For this review, take the finished solid that the model builds, in its own axes (mm). Face numbers are marked on the shaded views. Give positions to 0.01 mm unless a question says otherwise; leave off trailing zeros. Write each loop counter-clockwise with the first axis right and the second up, starting at its lowest first coordinate (ties: lowest second). Pieces come first, ordered by that corner, then holes. Notation, with made-up numbers: M 23,51 L 38,51 A21 ccw 38,76 Z; hole C 14,58 d3. An arc over 180 degrees is marked long. Write item = value, one per line.
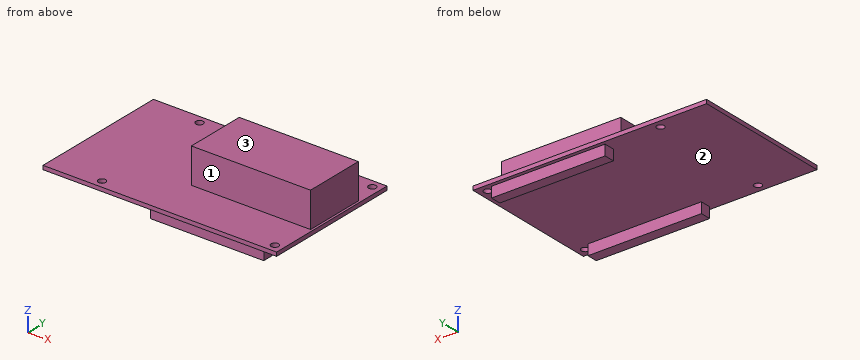
```python
from build123d import *

# Parameters (mm, degrees)
F0_W     = 100
F0_H     = 60
F0_R     = 1.6
F1_DEPTH = 1.65
F2_W     = 48.6
F2_H     = 4.5
F3_DEPTH = 4.5
F4_W     = 51
F4_H     = 26
F5_DEPTH = 15


with BuildPart() as f1:
    # F0 (on Top) → F1 (new body)
    with BuildSketch(Plane.XY):
        Rectangle(F0_W, F0_H)
        with Locations((-27.5, -26.5)):
            Circle(F0_R, mode=Mode.SUBTRACT)
        with Locations((46.5, -26.5)):
            Circle(F0_R, mode=Mode.SUBTRACT)
        with Locations((-27.5, 26.5)):
            Circle(F0_R, mode=Mode.SUBTRACT)
        with Locations((46.5, 26.5)):
            Circle(F0_R, mode=Mode.SUBTRACT)
    extrude(amount=F1_DEPTH)

    # F2 (on face) → F3 (join)
    with BuildSketch(Plane(origin=(0, 0, 0), x_dir=(1, 0, 0), z_dir=(0, 0, -1))):
        with Locations((19, 26.2)):
            Rectangle(F2_W, F2_H)
        with Locations((19, -26.2)):
            Rectangle(F2_W, F2_H)
    extrude(amount=F3_DEPTH)

    # F4 (on face) → F5 (join)
    with BuildSketch(Plane.XY.offset(1.65)):
        with Locations((23.5, 2.7)):
            Rectangle(F4_W, F4_H)
    extrude(amount=F5_DEPTH)


solid = f1.part
```
1. The part is to be moulded in two halves that separate along Y. For the marked faces 1, 2 and 3, say which applies: +Y half, -Y half, draft (parallel to the pull), parting line (faces both ways), or undercut.
Responses:
face_1 = -Y half
face_2 = undercut
face_3 = draft
2. We need section D-D, the plane x = 30. Write out the cut boundary in (y, z).
Responses:
outline = M -30,0 L -28.45,0 L -28.45,-4.5 L -23.95,-4.5 L -23.95,0 L 23.95,0 L 23.95,-4.5 L 28.45,-4.5 L 28.45,0 L 30,0 L 30,1.65 L 15.7,1.65 L 15.7,16.65 L -10.3,16.65 L -10.3,1.65 L -30,1.65 Z
3. We need section A-A, the plane x = 46.5. Write out the cut boundary in (y, z).
Responses:
outline = M -30,0 L -28.1,0 L -28.1,1.65 L -30,1.65 Z; M -24.9,0 L 24.9,0 L 24.9,1.65 L 15.7,1.65 L 15.7,16.65 L -10.3,16.65 L -10.3,1.65 L -24.9,1.65 Z; M 28.1,0 L 30,0 L 30,1.65 L 28.1,1.65 Z
4. For line 1 along Y through (x, z) = (-27.5, 0.45); line 2 along Z through (x, y) = (-13, -14); line 3 along Z through (x, y) = (33, -6.5), list the stretches that pass through material, from the lowest coordinate up. Write a range as from..to.
Responses:
line_1 = -30..-28.1, -24.9..24.9, 28.1..30
line_2 = 0..1.65
line_3 = 0..16.65
5. We need section B-B, the plane y = -26.5. Write out the cut boundary in (x, z).
Responses:
outline = M -50,0 L -29.1,0 L -29.1,1.65 L -50,1.65 Z; M -25.9,0 L -5.3,0 L -5.3,-4.5 L 43.3,-4.5 L 43.3,0 L 44.9,0 L 44.9,1.65 L -25.9,1.65 Z; M 48.1,0 L 50,0 L 50,1.65 L 48.1,1.65 Z
6. We need section C-C, the plane z = -1.25. Write out the cut boundary in (x, y).
Responses:
outline = M -5.3,-28.45 L 43.3,-28.45 L 43.3,-23.95 L -5.3,-23.95 Z; M -5.3,23.95 L 43.3,23.95 L 43.3,28.45 L -5.3,28.45 Z
7. Insertion check: P1, Ø3.5, axis at y = 25.5, z = -2.5, coming from the -X side; P2, Ø4.5, axis at x = 25, z = 10, coming from the -Y side; P3, Ø1.3, axis at x = 29.5, z = -2, coming from the -Y side. Each pin has a flat end and moves straight along its axis. Give the tip position at first contact, or say it passes through.
Responses:
P1 = -5.3
P2 = -10.3
P3 = -28.45
